Study the drawing (mm; zero at the part's minimum x, y, z) and answer. A direction names the side the tool comes from. Give positions to 0.01 mm unless a question says otherwise; leave off trailing zeros. Loops run counter-clockwise (first coordinate to the right, second up) from the corner with the lowest first, then second, coordinate; pieces in that order, holes last. Notation, with made-up numbers: (76.25, 58) - (80.25, 58) arc R20 ccw to (80.25, 64) - close; hole circle Ø1 at (75, -21). An arc over 180 degrees is marked (long way). Answer in a Markdown table with one row per item. Add a question column.
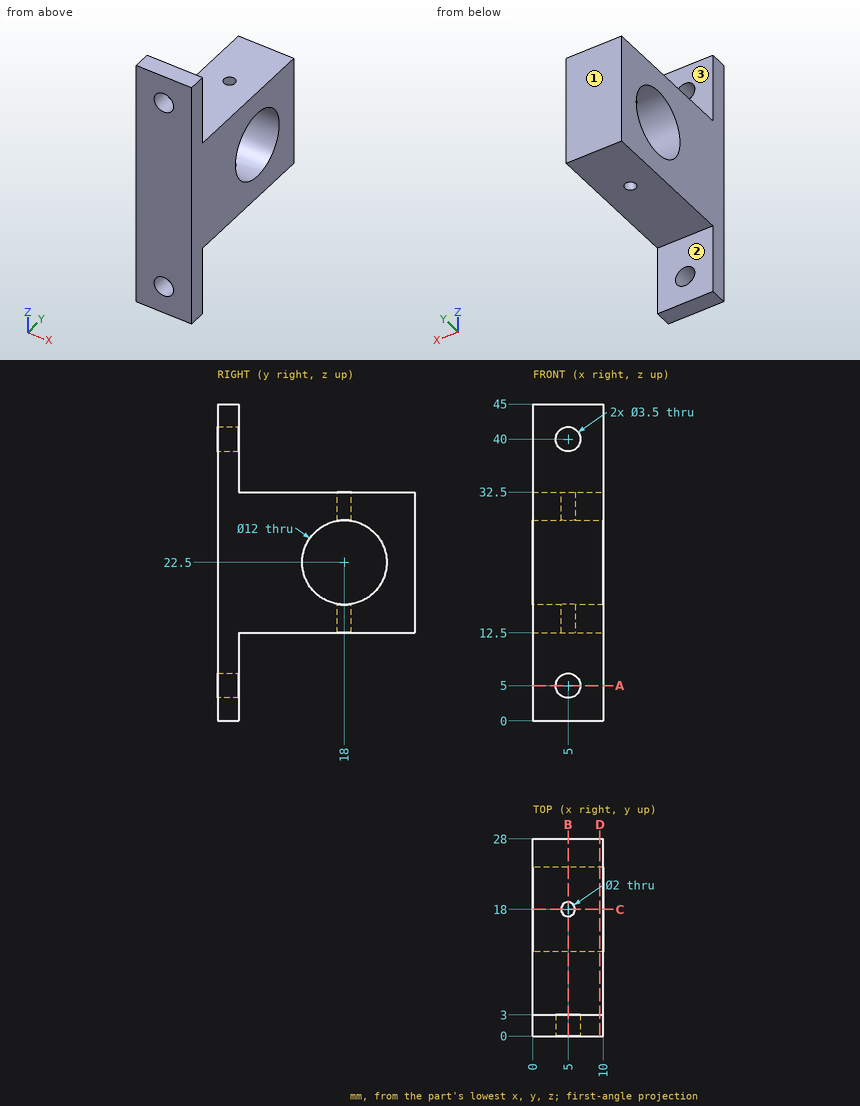
(1) Given pin 1 Ø1.6 at (x, y) = (5, 18) entering from -Z; pin 2 Ø5 at (x, z) = (6, 37.5) entering from +Y; pin 3 Ø2.5 at (x, y) = (5, 18) entering from -Z; pin 4 Ø4 at (x, y) = (3.5, 10.5) entering from +Z, each flat-ended and moving along its own axis, determine where each tip first touches the part or whether it passes through.
(2) A tool of negligible diameter and unlimited length cuts with its end or side. For the marked faces 1, 2 and 3, from which of +Z, -Z, +X, -X, +Y, -Y can it reach the whole face along a straight path? Write none if from no direction.
(3) A cutting plane is placed at C-C on y = 18. Determine the outline of the cut face in (x, z), plus the area to 3 significant figures.
(4) A cutting plane is placed at B-B on x = 5. Determine the outline of the cut face in (y, z).
(5) Find the intervals of material crossed by line 1 along X through (y, z) = (1.55, 40); line 2 along X through (y, z) = (18, 30.4); line 3 along Y through (x, z) = (6, 22.5), in increasing order. Write a range as [from, to].
(6) A cutting plane is placed at A-A on z = 5. Determine the outline of the cut face in (x, y).
(7) A cutting plane is placed at D-D on x = 9.5. Determine the outline of the cut face in (y, z).
Evaluation:
| question | item | result |
|---|---|---|
| 1 | pin 1 | passes through |
| 1 | pin 2 | stops at y = 3 |
| 1 | pin 3 | stops at z = 12.5 |
| 1 | pin 4 | stops at z = 32.5 |
| 2 | face 1 | +Z, -Z, +X, -X, +Y |
| 2 | face 2 | -Z, +X, -X, +Y |
| 2 | face 3 | +Z, +X, -X, +Y |
| 3 | outline | (0, 12.5) - (4, 12.5) - (4, 16.5) - (0, 16.5) - close; (0, 28.5) - (4, 28.5) - (4, 32.5) - (0, 32.5) - close; (6, 12.5) - (10, 12.5) - (10, 16.5) - (6, 16.5) - close; (6, 28.5) - (10, 28.5) - (10, 32.5) - (6, 32.5) - close |
| 3 | area | 64.0 mm² |
| 4 | outline | (0, 0) - (3, 0) - (3, 3.25) - (0, 3.25) - close; (0, 6.75) - (3, 6.75) - (3, 12.5) - (17, 12.5) - (17, 16.58) arc R6 cw to (17, 28.42) - (17, 32.5) - (3, 32.5) - (3, 38.25) - (0, 38.25) - close; (0, 41.75) - (3, 41.75) - (3, 45) - (0, 45) - close; (19, 12.5) - (28, 12.5) - (28, 32.5) - (19, 32.5) - (19, 28.42) arc R6 cw to (19, 16.58) - close |
| 5 | line 1 | x = [0, 3.25], [6.75, 10] |
| 5 | line 2 | x = [0, 4], [6, 10] |
| 5 | line 3 | y = [0, 12], [24, 28] |
| 6 | outline | (0, 0) - (3.25, 0) - (3.25, 3) - (0, 3) - close; (6.75, 0) - (10, 0) - (10, 3) - (6.75, 3) - close |
| 7 | outline | (0, 0) - (3, 0) - (3, 12.5) - (28, 12.5) - (28, 32.5) - (3, 32.5) - (3, 45) - (0, 45) - close; hole circle Ø12 at (18, 22.5) |
